Geometry: final body of the model. Coordinates: model frame, mm. A direction names the side the tool comes from. Round coordinates to 2 decimals unless told otherwise and drop trailing zeros. Order: outer loops, then holes, each group sorted by start corner. A loop starts at its lowest first (then second) coordinate and runs counter-clockwise, first axis right, second up. Notation, with made-up numbers: (27, 61.5) -> (62, 61.5) arc R27 cw to (62, 78.5) -> close; hole circle Ø11 at (7, 6.25). An arc over 180 degrees is marked (long way). Put each result on its own line as item: value.
```python
from build123d import *

# Parameters (mm, degrees)
BOX016_W     = 9
BOX016_H     = 13
BOX016_DEPTH = 60
BOX004_W     = 9
BOX004_H     = 13
BOX004_DEPTH = 60
BOX005_W     = 9
BOX005_H     = 13
BOX005_DEPTH = 60
BOX006_W     = 9
BOX006_H     = 13
BOX006_DEPTH = 60
BOX007_W     = 9
BOX007_H     = 13
BOX007_DEPTH = 60
BOX008_W     = 9
BOX008_H     = 13
BOX008_DEPTH = 60
BOX009_W     = 9
BOX009_H     = 13
BOX009_DEPTH = 60
BOX010_W     = 9
BOX010_H     = 13
BOX010_DEPTH = 60
BOX011_W     = 9
BOX011_H     = 13
BOX011_DEPTH = 60
BOX012_W     = 9
BOX012_H     = 13
BOX012_DEPTH = 60
BOX013_W     = 9
BOX013_H     = 13
BOX013_DEPTH = 60
BOX014_W     = 9
BOX014_H     = 13
BOX014_DEPTH = 60
BOX015_W     = 9
BOX015_H     = 13
BOX015_DEPTH = 60
BOX017_W     = 9
BOX017_H     = 13
BOX017_DEPTH = 60
BOX018_W     = 9
BOX018_H     = 13
BOX018_DEPTH = 60
BOX019_W     = 9
BOX019_H     = 13
BOX019_DEPTH = 60
BOX020_W     = 9
BOX020_H     = 13
BOX020_DEPTH = 60
BOX003_W     = 9
BOX003_H     = 13
BOX003_DEPTH = 60
BOX002_W     = 200
BOX002_H     = 15
BOX002_DEPTH = 60
FILLET_R     = 8


with BuildPart() as cube016:
    # Box016 → Box016 (new body)
    with BuildSketch(Plane(origin=(145, -15, 0), x_dir=(1, 0, 0), z_dir=(0, 0, 1))):
        with Locations((4.5, 6.5)):
            Rectangle(BOX016_W, BOX016_H)
    extrude(amount=BOX016_DEPTH)


with BuildPart() as cube004:
    # Box004 → Box004 (new body)
    with BuildSketch(Plane(origin=(13, -15, 0), x_dir=(1, 0, 0), z_dir=(0, 0, 1))):
        with Locations((4.5, 6.5)):
            Rectangle(BOX004_W, BOX004_H)
    extrude(amount=BOX004_DEPTH)


with BuildPart() as cube005:
    # Box005 → Box005 (new body)
    with BuildSketch(Plane(origin=(24, -15, 0), x_dir=(1, 0, 0), z_dir=(0, 0, 1))):
        with Locations((4.5, 6.5)):
            Rectangle(BOX005_W, BOX005_H)
    extrude(amount=BOX005_DEPTH)


with BuildPart() as cube006:
    # Box006 → Box006 (new body)
    with BuildSketch(Plane(origin=(35, -15, 0), x_dir=(1, 0, 0), z_dir=(0, 0, 1))):
        with Locations((4.5, 6.5)):
            Rectangle(BOX006_W, BOX006_H)
    extrude(amount=BOX006_DEPTH)


with BuildPart() as cube007:
    # Box007 → Box007 (new body)
    with BuildSketch(Plane(origin=(46, -15, 0), x_dir=(1, 0, 0), z_dir=(0, 0, 1))):
        with Locations((4.5, 6.5)):
            Rectangle(BOX007_W, BOX007_H)
    extrude(amount=BOX007_DEPTH)


with BuildPart() as cube008:
    # Box008 → Box008 (new body)
    with BuildSketch(Plane(origin=(57, -15, 0), x_dir=(1, 0, 0), z_dir=(0, 0, 1))):
        with Locations((4.5, 6.5)):
            Rectangle(BOX008_W, BOX008_H)
    extrude(amount=BOX008_DEPTH)


with BuildPart() as cube009:
    # Box009 → Box009 (new body)
    with BuildSketch(Plane(origin=(68, -15, 0), x_dir=(1, 0, 0), z_dir=(0, 0, 1))):
        with Locations((4.5, 6.5)):
            Rectangle(BOX009_W, BOX009_H)
    extrude(amount=BOX009_DEPTH)


with BuildPart() as cube010:
    # Box010 → Box010 (new body)
    with BuildSketch(Plane(origin=(79, -15, 0), x_dir=(1, 0, 0), z_dir=(0, 0, 1))):
        with Locations((4.5, 6.5)):
            Rectangle(BOX010_W, BOX010_H)
    extrude(amount=BOX010_DEPTH)


with BuildPart() as cube011:
    # Box011 → Box011 (new body)
    with BuildSketch(Plane(origin=(90, -15, 0), x_dir=(1, 0, 0), z_dir=(0, 0, 1))):
        with Locations((4.5, 6.5)):
            Rectangle(BOX011_W, BOX011_H)
    extrude(amount=BOX011_DEPTH)


with BuildPart() as cube012:
    # Box012 → Box012 (new body)
    with BuildSketch(Plane(origin=(101, -15, 0), x_dir=(1, 0, 0), z_dir=(0, 0, 1))):
        with Locations((4.5, 6.5)):
            Rectangle(BOX012_W, BOX012_H)
    extrude(amount=BOX012_DEPTH)


with BuildPart() as cube013:
    # Box013 → Box013 (new body)
    with BuildSketch(Plane(origin=(112, -15, 0), x_dir=(1, 0, 0), z_dir=(0, 0, 1))):
        with Locations((4.5, 6.5)):
            Rectangle(BOX013_W, BOX013_H)
    extrude(amount=BOX013_DEPTH)


with BuildPart() as cube014:
    # Box014 → Box014 (new body)
    with BuildSketch(Plane(origin=(123, -15, 0), x_dir=(1, 0, 0), z_dir=(0, 0, 1))):
        with Locations((4.5, 6.5)):
            Rectangle(BOX014_W, BOX014_H)
    extrude(amount=BOX014_DEPTH)


with BuildPart() as cube015:
    # Box015 → Box015 (new body)
    with BuildSketch(Plane(origin=(134, -15, 0), x_dir=(1, 0, 0), z_dir=(0, 0, 1))):
        with Locations((4.5, 6.5)):
            Rectangle(BOX015_W, BOX015_H)
    extrude(amount=BOX015_DEPTH)


with BuildPart() as cube017:
    # Box017 → Box017 (new body)
    with BuildSketch(Plane(origin=(156, -15, 0), x_dir=(1, 0, 0), z_dir=(0, 0, 1))):
        with Locations((4.5, 6.5)):
            Rectangle(BOX017_W, BOX017_H)
    extrude(amount=BOX017_DEPTH)


with BuildPart() as cube018:
    # Box018 → Box018 (new body)
    with BuildSketch(Plane(origin=(167, -15, 0), x_dir=(1, 0, 0), z_dir=(0, 0, 1))):
        with Locations((4.5, 6.5)):
            Rectangle(BOX018_W, BOX018_H)
    extrude(amount=BOX018_DEPTH)


with BuildPart() as cube019:
    # Box019 → Box019 (new body)
    with BuildSketch(Plane(origin=(178, -15, 0), x_dir=(1, 0, 0), z_dir=(0, 0, 1))):
        with Locations((4.5, 6.5)):
            Rectangle(BOX019_W, BOX019_H)
    extrude(amount=BOX019_DEPTH)


with BuildPart() as cube020:
    # Box020 → Box020 (new body)
    with BuildSketch(Plane(origin=(189, -15, 0), x_dir=(1, 0, 0), z_dir=(0, 0, 1))):
        with Locations((4.5, 6.5)):
            Rectangle(BOX020_W, BOX020_H)
    extrude(amount=BOX020_DEPTH)


with BuildPart() as compound:
    # Box003 → Box003 (new body)
    with BuildSketch(Plane(origin=(2, -15, 0), x_dir=(1, 0, 0), z_dir=(0, 0, 1))):
        with Locations((4.5, 6.5)):
            Rectangle(BOX003_W, BOX003_H)
    extrude(amount=BOX003_DEPTH)

    # Compound: union Cube016, Cube004, Cube005, Cube006, Cube007, Cube008, Cube009, Cube010, Cube011, Cube012, Cube013, Cube014, Cube015, Cube017, Cube018, Cube019, Cube020
    add(cube016.part)
    add(cube004.part)
    add(cube005.part)
    add(cube006.part)
    add(cube007.part)
    add(cube008.part)
    add(cube009.part)
    add(cube010.part)
    add(cube011.part)
    add(cube012.part)
    add(cube013.part)
    add(cube014.part)
    add(cube015.part)
    add(cube017.part)
    add(cube018.part)
    add(cube019.part)
    add(cube020.part)


with BuildPart() as left_heatsink:
    # Box002 → Box002 (new body)
    with BuildSketch(Plane(origin=(0, -15, 0), x_dir=(1, 0, 0), z_dir=(0, 0, 1))):
        with Locations((100, 7.5)):
            Rectangle(BOX002_W, BOX002_H)
    extrude(amount=BOX002_DEPTH)

    # Cut001: cut Compound
    add(compound.part, mode=Mode.SUBTRACT)

    # Fillet
    fillet_edges = [left_heatsink.edges().sort_by_distance(p)[0] for p in [
        (1, -15, 0),
        (1, -15, 60),
        (199, -15, 60),
        (188, -15, 60),
        (177, -15, 60),
        (166, -15, 60),
        (155, -15, 60),
        (144, -15, 60),
        (133, -15, 60),
        (122, -15, 60),
        (111, -15, 60),
        (100, -15, 60),
        (89, -15, 60),
        (78, -15, 60),
        (67, -15, 60),
        (56, -15, 60),
        (45, -15, 60),
        (34, -15, 60),
        (23, -15, 60),
        (12, -15, 60),
        (199, -15, 0),
        (188, -15, 0),
        (177, -15, 0),
        (166, -15, 0),
        (155, -15, 0),
        (144, -15, 0),
        (133, -15, 0),
        (122, -15, 0),
        (111, -15, 0),
        (100, -15, 0),
        (89, -15, 0),
        (78, -15, 0),
        (67, -15, 0),
        (56, -15, 0),
        (45, -15, 0),
        (34, -15, 0),
        (23, -15, 0),
        (12, -15, 0),
    ]]
    fillet(fillet_edges, radius=FILLET_R)


solid = left_heatsink.part
```
1. Material intervals for probe 1 along Y at (x, z) = (146.5, 43); probe 2 along Z at (x, y) = (89.5, -7.5); probe 3 along Z at (x, y) = (188, -13.25), sorted ascending.
Ans:
probe 1: -2 to 0
probe 2: 0.02 to 59.98
probe 3: 3.01 to 56.99
2. Set-up query: faces 5 (the face through (79, -9, 30)), 6 (the face through (100.014, -12.594, 57.719)). Return all of +Z, -Z, +X, -X, +Y, -Y with unobstructed straight access to the full face (end or side cutting, diameter ignored); none if empty.
Ans:
face 5: +Z, -Z, -Y
face 6: +Z, +X, -X, -Y
3. Contact query for a flat-ended pin moving along its axis: P1, Ø1, axis at x = 150.5, z = 38.5, coming from the -Y side. Output: stop coordinate, or through.
Ans:
P1: y = -2
4. Cut plane B-B on x = 26.5. Return loops of the section in (y, z).
Ans:
outline: (-2, 0) -> (0, 0) -> (0, 60) -> (-2, 60) -> close
5. Draft query along X for faces 1 (the face through (200, -8, 30)), 2 (the face through (45.014, -12.594, 2.281)), 3 (the face through (198, -9, 30)), 4 (the face through (28, -2, 30)). Return one class per face: +X half, -X half, draft (parallel to the pull), parting line (faces both ways), or undercut.
Ans:
face 1: +X half
face 2: draft
face 3: undercut
face 4: undercut
6. Cut plane A-A on y = -4.75. State how many separate pieces and enclosed holes the cut face has, and give its area (3 significant figures).
Ans:
separate pieces: 19
enclosed holes: 0
area: 2,280 mm²
